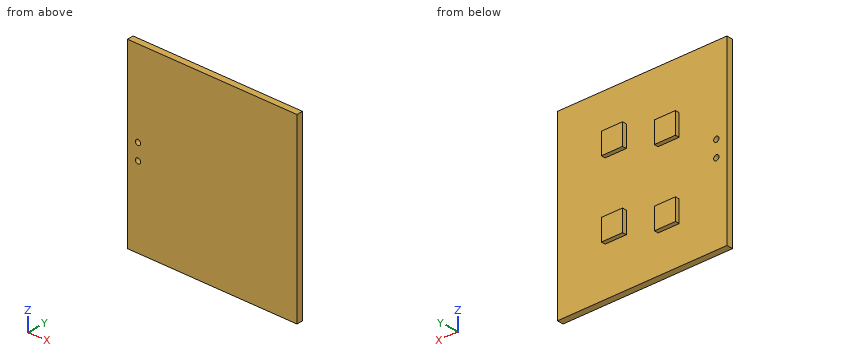
```python
from build123d import *

# Parameters (mm, degrees)
SKETCH2_W           = 40.64
SKETCH2_H           = 43.18
BOSS_EXTRUDE1_DEPTH = 1.524
SKETCH3_R           = 0.635
CUT_EXTRUDE1_DEPTH  = 60.316478115
SKETCH4_W           = 5.08
SKETCH4_H           = 5.08
BOSS_EXTRUDE2_DEPTH = 1.016


with BuildPart() as part:
    # Sketch2 → Boss-Extrude1 (new body)
    with BuildSketch(Plane(origin=(0, 0, 0), x_dir=(1, 0, 0), z_dir=(0, 1, 0))):
        with Locations((20.32, 21.59)):
            Rectangle(SKETCH2_W, SKETCH2_H)
    extrude(amount=BOSS_EXTRUDE1_DEPTH)

    # Sketch3 → Cut-Extrude1 (cut, through all)
    with BuildSketch(Plane(origin=(0, 1.524, 0), x_dir=(1, 0, 0), z_dir=(0, 1, 0))):
        with Locations(Location((2.54, 24.13, 0), (0, 0, 270))):
            Circle(SKETCH3_R)
        with Locations(Location((2.54, 20.32, 0), (0, 0, 270))):
            Circle(SKETCH3_R)
    extrude(amount=-CUT_EXTRUDE1_DEPTH, mode=Mode.SUBTRACT)

    # Sketch4 → Boss-Extrude2 (add)
    with BuildSketch(Plane(origin=(0, 1.524, 0), x_dir=(1, 0, 0), z_dir=(0, 1, 0))):
        with Locations((13.97, 31.75)):
            Rectangle(SKETCH4_W, SKETCH4_H)
        with Locations((26.67, 29.21)):
            Rectangle(SKETCH4_W, SKETCH4_H)
        with Locations((13.97, 13.97)):
            Rectangle(SKETCH4_W, SKETCH4_H)
        with Locations((26.67, 11.43)):
            Rectangle(SKETCH4_W, SKETCH4_H)
    extrude(amount=BOSS_EXTRUDE2_DEPTH)


solid = part.part
```
Read the model definition and answer for the solid it produces. Units are mm, in the model's axes. Coordinates: 2 decimals unless noted, no trailing zeros. Loops run counter-clockwise (first coordinate to the right, second up) from the corner with the lowest first, then second, coordinate; pieces in that order, holes last. Notation, with made-up numbers: (86, 70.25) - (119, 70.25) arc R16 ccw to (119, 90.25) - close; hole circle Ø1 at (10, 85.5). An arc over 180 degrees is marked (long way). Answer in a Markdown table with one row per item.
1. Find section A-A, the plane z = -24.13. Write down the section's boundary in (x, y) (3 decimals).
Conclusion:
| item | result |
|---|---|
| outline | (0, 0) - (1.905, 0) - (1.905, 1.524) - (0, 1.524) - close; (3.175, 0) - (40.64, 0) - (40.64, 1.524) - (3.175, 1.524) - close |
2. Find section C-C, the plane x = 31. Write down the section's boundary in (y, z), then the cut area to 3 significant figures.
Conclusion:
| item | result |
|---|---|
| outline | (0, -43.18) - (1.52, -43.18) - (1.52, 0) - (0, 0) - close |
| area | 65.8 mm² |
3. Given pin 1 (12 mm diameter, centred on x = 32, z = -6.5, fed in from -Y); pin 2 (1 mm diameter, centred on x = 2.54, z = -20.32, fed in from +Y); pin 3 (0.8 mm diameter, centred on x = 13.5, y = 2, fed in from +Z); pin 4 (0.8 mm diameter, centred on y = 2.5, z = -12, fed in from -X), each flat-ended and moving along its own axis, determine where each tip first touches the part or whether it passes through.
Conclusion:
| item | result |
|---|---|
| pin 1 | stops at y = 0 |
| pin 2 | passes through |
| pin 3 | stops at z = -11.43 |
| pin 4 | stops at x = 11.43 |
4. Straight lines are drawn through the part: line 1 (X direction, y = 1.2, z = -24.13) (3 decimals); line 2 (Y direction, x = 13, z = -21.5); line 3 (Z direction, x = 2, y = 1.3). For each, find the intervals that lie inside material, in ascending order.
Conclusion:
| item | result |
|---|---|
| line 1 | x = 0 to 1.905, 3.175 to 40.64 |
| line 2 | y = 0 to 1.52 |
| line 3 | z = -43.18 to -24.46, -23.8 to -20.65, -19.99 to 0 |
5. Find section B-B, the plane x = 2.54. Write down the section's boundary in (y, z) (3 decimals), then the cut area to 3 significant figures.
Conclusion:
| item | result |
|---|---|
| outline | (0, -43.18) - (1.524, -43.18) - (1.524, -24.765) - (0, -24.765) - close; (0, -23.495) - (1.524, -23.495) - (1.524, -20.955) - (0, -20.955) - close; (0, -19.685) - (1.524, -19.685) - (1.524, 0) - (0, 0) - close |
| area | 61.9 mm² |
